Here's how the part is built. I have some questions about the finished solid (model axes, mm). A direction names the side the tool comes from. Give positions to 0.01 mm unless a question says otherwise; leave off trailing zeros. Write each loop counter-clockwise with the first axis right and the second up, starting at its lowest first coordinate (ties: lowest second). Pieces come first, ordered by that corner, then holes. Notation, with made-up numbers: (-7, 45.5) - (21, 45.5) arc R17 cw to (21, 56.5) - close; hole circle Ø3 at (-20.5, 32.5). An arc over 180 degrees is marked (long way). One line per item, written item: value. Start each with the question number.
1) On a 3-axis mill with a long thin cutter (end or side, diameter ignored), from which of +Z, -Z, +X, -X, +Y, -Y can I reach the whole of each face in a straight line? I mean faces 1 (the flat face through (12.74, 88.74, 3.45)), 2 (the cylindrical face through (64.662, 26.81, 9.86)). Say none if no direction works.
2) Imagine slicing it at C-C on y = 53. Write out the boundary of the cut face in (x, z).
3) Please list where these lines run through material, in increasing order: L1, parallel to Z at x = 13.5, y = -73; L2, parallel to Y at x = -1.5, z = 10.75; L3, parallel to X at y = -57, z = 8.75. Write a range as [from, to].
4) Imagine slicing it at B-B on z = 16. Write out the boundary of the cut face in (x, y).
5) Imagine slicing it at D-D on x = 41. Write out the boundary of the cut face in (y, z), plus the area to 3 significant figures.
6) I'm going to push flat-ended pins straight in: P1, Ø12, axis at y = -35, z = 2, coming from the -X side; P2, Ø8, axis at y = 17.5, z = 2.5, coming from the -X side; P3, Ø2, axis at x = 14, y = -58, coming from the -Z side; P4, Ø1.5, axis at x = -2.5, z = 14.5, coming from the -Y side. Where does each tip first touch, or does it pass through?
7) Imagine slicing it at A-A on x = 0. Write out the boundary of the cut face in (y, z).
Autodesk Inventor part; units mm, degrees
ref_plane "YZ Plane" through (0, 0, 0) normal (1, 0, 0) x (0, 1, 0)
ref_plane "XZ Plane" through (0, 0, 0) normal (0, 1, 0) x (-1, 0, 0)
ref_plane "XY Plane" through (0, 0, 0) normal (0, 0, 1) x (1, 0, 0)
sketch "Skizze2" plane through (0, 0, 0) normal (0, 0, 1) x (1, 0, 0)
  line L0 (-117.4666, 197.4366) -> (107.72, 197.4366) construction
  line L1 (107.72, 197.4366) -> (107.72, -200.7323) construction
  line L2 (107.72, -200.7323) -> (-117.4666, -200.7323) construction
  line L3 (-117.4666, -200.7323) -> (-117.4666, 197.4366) construction
  circle A0 centre (0, 0) radius 70
  line L4 (-20.6981, 66.87) -> (-5, 110)
  line L5 (-5, 110) -> (5, 110)
  line L6 (5, 110) -> (20.6981, 66.87)
  line L7 (-20.6981, -66.87) -> (-5, -110)
  line L8 (-5, -110) -> (5, -110)
  line L9 (5, -110) -> (20.6981, -66.87)
  line L10 (0, 110) -> (0, 0)
  line L11 (0, 0) -> (0, -110)
  dimension "d3" = 110
  dimension "d4" = 110
  dimension "d5" = 110
  dimension "d8" = 140
  dimension "d9" = 110
  dimension "d10" = 110
  dimension "d11" = 110
  dimension "d12" = 10
  dimension "d13" = 10
extrude "Extrusion1" add sketch "Skizze2" along normal blind 20 contours A0 L11 L10 | L10 L11 A0
extrude "Extrusion2" add sketch "Skizze2" along normal blind 7 contours A0 L10 L5 L6 | L9 L8 L11 A0 | A0 L4 L5 L10 | L11 L8 L7 A0
sketch "Skizze3" plane through (0, 0, 20) normal (0, 0, 1) x (1, 0, 0)
  line L0 (-65, 65) -> (65, 65) construction
  line L1 (65, 65) -> (65, -65.4377) construction
  line L2 (65, -65.4377) -> (-65, -65.4377) construction
  line L3 (-65, -65.4377) -> (-65, 65) construction
  point P0 (0, 0)
properties part number "waage" material "PC/ABS-Kunststoff, 3DDruck, PLA"
Numbers:
1. face 1: +Z, -Z, +X, +Y
1. face 2: +Z
2. outline: (-45.73, 0) - (45.73, 0) - (45.73, 20) - (-45.73, 20) - close
3. L1: [0, 7]
3. L2: [-69.98, 69.98]
3. L3: [-40.63, 40.63]
4. outline: circle Ø140 at (0, 0)
5. outline: (-56.74, 0) - (56.74, 0) - (56.74, 20) - (-56.74, 20) - close
5. area: 2,270 mm^2
6. P1: x = -63.71
6. P2: x = -68.69
6. P3: z = 0
6. P4: y = -69.98
7. outline: (-110, 0) - (110, 0) - (110, 7) - (70, 7) - (70, 20) - (-70, 20) - (-70, 7) - (-110, 7) - close
